from build123d import *

# Parameters (mm, degrees)
SKETCH1_W           = 10
SKETCH1_H           = 45.3
BOSS_EXTRUDE2_DEPTH = 2
SKETCH2_W           = 3
SKETCH2_H           = 3
BOSS_EXTRUDE3_DEPTH = 22
SKETCH3_R           = 1
CUT_EXTRUDE1_DEPTH  = 22
SKETCH4_R           = 1
CUT_EXTRUDE2_DEPTH  = 22


with BuildPart() as part:
    # Sketch1 → Boss-Extrude2 (new body)
    with BuildSketch(Plane.XY):
        with Locations((2.593477414, 6.123019747)):
            Rectangle(SKETCH1_W, SKETCH1_H)
    extrude(amount=BOSS_EXTRUDE2_DEPTH)

    # Sketch2 → Boss-Extrude3 (add)
    with BuildSketch(Plane(origin=(0, 0, 0), x_dir=(-1, 0, 0), z_dir=(0, 0, -1))):
        with Locations((0.906522586, 27.273019747)):
            Rectangle(SKETCH2_W, SKETCH2_H)
        with Locations((0.906522586, -15.026980253)):
            Rectangle(SKETCH2_W, SKETCH2_H)
    extrude(amount=BOSS_EXTRUDE3_DEPTH)

    # Sketch3 → Cut-Extrude1 (cut)
    with BuildSketch(Plane.ZY.offset(2.406522586)):
        with Locations((-19.5, 27.273019747)):
            Circle(SKETCH3_R)
        with Locations((-1, 27.273019747)):
            Circle(SKETCH3_R)
        with Locations((-1, -15.026980253)):
            Circle(SKETCH3_R)
        with Locations((-19.5, -15.026980253)):
            Circle(SKETCH3_R)
    extrude(amount=-CUT_EXTRUDE1_DEPTH, mode=Mode.SUBTRACT)

    # Sketch4 → Cut-Extrude2 (cut)
    with BuildSketch(Plane(origin=(0, 0, 0), x_dir=(-1, 0, 0), z_dir=(0, 0, -1))):
        with Locations((-2.593477414, 6.073019747)):
            Circle(SKETCH4_R)
    extrude(amount=-CUT_EXTRUDE2_DEPTH, mode=Mode.SUBTRACT)


solid = part.part
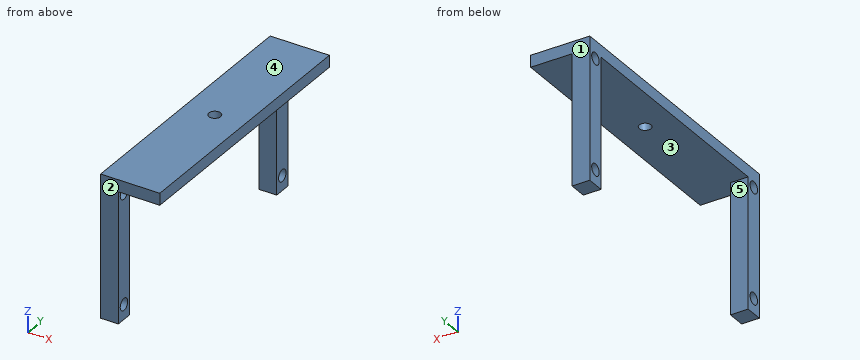
Read the model definition and answer for the solid it produces. Units are mm, in the model's axes. Face numbers are marked on the shaded views. A direction names the side the tool comes from. Round coordinates to 2 decimals unless told otherwise and drop trailing zeros. Loops run counter-clockwise (first coordinate to the right, second up) from the corner with the lowest first, then second, coordinate; pieces in that order, holes last. Notation, with made-up numbers: (65.5, -23) - (115.5, -23) arc R15 ccw to (115.5, -6) - close; hole circle Ø8 at (89.5, -10). An arc over 180 degrees is marked (long way). One line per question, with ' | ' between items. Start each with the question number.
Q1. Section D-D on y = 19 is taken. Give the vertices of the cut face in (x, z), plus the area to 3 significant figures.
Q2. For a pull along Y with two mould halves and no side action, classify the marked faces 1, 2 and 3 as +Y half, -Y half, draft (parallel to the pull), parting line (faces both ways), or undercut.
Q3. Section B-B on z = -7 is taken. Give the vertices of the cut face in (x, y), plus the area to 3 significant figures.
Q4. Find the intervals of material crossed by L1, parallel to Y at x = -1.3, z = -19.5; L2, parallel to Y at x = -1.5, z = -8.75; L3, parallel to Z at x = 0.5, y = 7, in increasing order.
Q5. For the marked faces 4 and 5, determine the directions among +Z, -Z, +X, -X, +Y, -Y from which every point of the face is accessible in a straight line to the end or side of a thin tool.
Q6. Flat-ended cylindrical pins translate along their axes: pin 1 (3 mm diameter, centred on y = -15.03, z = -19.5, fed in from +X); pin 2 (5 mm diameter, centred on x = 2.5, y = 17, fed in from -Z). Find the tip coordinate at first contact, or state that the pin passes through.
Q7. Section C-C on x = -0.5 is taken. Give the vertices of the cut face in (y, z), plus the area to 3 significant figures.
Q8. Section A-A on z = -19.5 is taken. Give the vertices of the cut face in (x, y).
Established:
1) outline: (-2.41, 0) - (7.59, 0) - (7.59, 2) - (-2.41, 2) - close | area: 20.0 mm²
2) face 1: +Y half | face 2: -Y half | face 3: undercut
3) outline: (-2.41, -16.53) - (0.59, -16.53) - (0.59, -13.53) - (-2.41, -13.53) - close; (-2.41, 25.77) - (0.59, 25.77) - (0.59, 28.77) - (-2.41, 28.77) - close | area: 18.0 mm²
4) L1: -16.53 to -16.03, -14.03 to -13.53, 25.77 to 26.27, 28.27 to 28.77 | L2: -16.53 to -13.53, 25.77 to 28.77 | L3: 0 to 2
5) face 4: +Z, +X, -X, +Y, -Y | face 5: -Z, +X, -X
6) pin 1: x = 0.59 | pin 2: z = 0
7) outline: (-16.53, -22) - (-13.53, -22) - (-13.53, 0) - (25.77, 0) - (25.77, -22) - (28.77, -22) - (28.77, 2) - (-16.53, 2) - close; hole circle Ø2 at (-15.03, -19.5); hole circle Ø2 at (-15.03, -1); hole circle Ø2 at (27.27, -19.5); hole circle Ø2 at (27.27, -1) | area: 210 mm²
8) outline: (-2.41, -16.53) - (0.59, -16.53) - (0.59, -16.03) - (-2.41, -16.03) - close; (-2.41, -14.03) - (0.59, -14.03) - (0.59, -13.53) - (-2.41, -13.53) - close; (-2.41, 25.77) - (0.59, 25.77) - (0.59, 26.27) - (-2.41, 26.27) - close; (-2.41, 28.27) - (0.59, 28.27) - (0.59, 28.77) - (-2.41, 28.77) - close
